```python
from build123d import *

# Parameters (mm, degrees)
F0_W     = 400
F0_H     = 200
F1_DEPTH = 10
F2_R     = 12.5
F3_DEPTH = 200
F4_R     = 12.5
F5_DEPTH = 200


with BuildPart() as f1:
    # F0 (on Front) → F1 (new body)
    with BuildSketch(Plane.XZ):
        with Locations((-15.897054, -26.061756)):
            Rectangle(F0_W, F0_H)
    extrude(amount=F1_DEPTH)

    # F2 (on Front) → F3 (join)
    with BuildSketch(Plane.XZ):
        with Locations((-195.897054, 53.938244)):
            Circle(F2_R)
    extrude(amount=-F3_DEPTH)

    # F4 (on face) → F5 (join)
    with BuildSketch(Plane(origin=(0, 0, 0), x_dir=(-1, 0, 0), z_dir=(0, 1, 0))):
        with Locations((-164.102946, 53.938244)):
            Circle(F4_R)
        with Locations((-164.102946, -106.061756)):
            Circle(F4_R)
        with Locations((195.897054, -106.061756)):
            Circle(F4_R)
    extrude(amount=F5_DEPTH)


solid = f1.part
```
Geometry check sheet. Reference: the model listing, model coordinates, mm. A direction names the side the tool comes from. Round coordinates to 2 decimals unless told otherwise and drop trailing zeros. Loops run counter-clockwise (first coordinate to the right, second up) from the corner with the lowest first, then second, coordinate; pieces in that order, holes last. Notation, with made-up numbers: (36.5, 16.5) - (87.5, 16.5) arc R29 cw to (87.5, 54.5) - close; hole circle Ø2 at (44.5, -8). An arc over 180 degrees is marked (long way). Use a Markdown table: item, result.
Q1. Access from +Z, -Z, +X, -X, +Y, -Y to the whole of each face (thin tool, end or side, straight path). Record for faces 5 (the cylindrical face through (-205.1, 98.6, 62.4)), 6 (the flat face through (-19, -10, -25)).
Solutions:
| item | result |
|---|---|
| face 5 | +Y |
| face 6 | +Z, -Z, +X, -X, -Y |
Q2. Cross-section at D-D on z = -17. Record the cut outline in (x, y).
Solutions:
| item | result |
|---|---|
| outline | (-215.9, -10) - (184.1, -10) - (184.1, 0) - (-215.9, 0) - close |
Q3. Go/stop test with a flat-tipped pin: P1, Ø5, axis at y = 133.5, z = 52.5, coming from the +X side. Record where the tip stops, or that it passes through.
Solutions:
| item | result |
|---|---|
| P1 | stops at x = 176.6 |
Q4. Draft check along Z on faces 1 (the flat face through (-19, -5, -126.062)), 2 (the cylindrical face through (-186.684, 98.6, -97.614)), 3 (the cylindrical face through (152.18, 98.6, -102.31)), 4 (the flat face through (164, 200, -106)). Enter one of: released by +Z, released by -Z, zero draft, split by the parting line, or undercut.
Solutions:
| item | result |
|---|---|
| face 1 | released by -Z |
| face 2 | undercut |
| face 3 | undercut |
| face 4 | zero draft |
Q5. Cross-section at B-B on x = 147.5. Record the cut outline in (y, z).
Solutions:
| item | result |
|---|---|
| outline | (-10, -126.06) - (0, -126.06) - (0, 73.94) - (-10, 73.94) - close |
Q6. Cross-section at C-C on y = 176.5. Record the cut outline in (x, z), plus the area to 3 significant figures.
Solutions:
| item | result |
|---|---|
| outline | circle Ø25 at (-195.9, -106.06); circle Ø25 at (-195.9, 53.94); circle Ø25 at (164.1, -106.06); circle Ø25 at (164.1, 53.94) |
| area | 1,960 mm2 |
Q7. Cross-section at A-A on z = -98. Record the cut outline in (x, y), plus the area to 3 significant figures.
Solutions:
| item | result |
|---|---|
| outline | (-215.9, -10) - (184.1, -10) - (184.1, 0) - (173.66, 0) - (173.66, 200) - (154.55, 200) - (154.55, 0) - (-186.34, 0) - (-186.34, 200) - (-205.45, 200) - (-205.45, 0) - (-215.9, 0) - close |
| area | 11,600 mm2 |
Q8. Material ranges on line 1 (Y direction, x = 1.5, z = -49); line 2 (X direction, y = 114, z = 48.5); line 3 (X direction, y = 72, z = -100.5), recorded low to high.
Solutions:
| item | result |
|---|---|
| line 1 | y = -10 to 0 |
| line 2 | x = -207.15 to -184.64, 152.85 to 175.36 |
| line 3 | x = -207.09 to -184.7, 152.91 to 175.3 |
